from build123d import *

# Parameters (mm, degrees)
SKETCH1_R           = 11
SKETCH1_R_2         = 1.25
BOSS_EXTRUDE1_DEPTH = 3.175


with BuildPart() as part:
    # Sketch1 → Boss-Extrude1 (new body)
    with BuildSketch(Plane(origin=(0, 0, 0), x_dir=(0, 0, -1), z_dir=(1, 0, 0))):
        Circle(SKETCH1_R)
        with BuildLine():
            Line((-2.5, -1.658312395), (-2.5, 1.658312395))
            ThreePointArc((-2.5, 1.658312395), (0.866025404, 2.872281323), (3, 0))
            ThreePointArc((3, 0), (0.866025404, -2.872281323), (-2.5, -1.658312395))
        make_face(mode=Mode.SUBTRACT)
        with Locations((-8, 0)):
            Circle(SKETCH1_R_2, mode=Mode.SUBTRACT)
        with Locations((8, 0)):
            Circle(SKETCH1_R_2, mode=Mode.SUBTRACT)
    extrude(amount=BOSS_EXTRUDE1_DEPTH)


solid = part.part
The model under review builds one solid part; all positions refer to its coordinate system, in mm. Round coordinates to 2 decimals unless told otherwise and drop trailing zeros. Order: outer loops, then holes, each group sorted by start corner. A loop starts at its lowest first (then second) coordinate and runs counter-clockwise, first axis right, second up. Notation, with made-up numbers: (67, 71) -> (77, 71) arc R26 cw to (77, 93) -> close; hole circle Ø3 at (-15.75, -6). An arc over 180 degrees is marked (long way). Write item = value, one per line. Start each with the question number.
Item 1: Consider section C-C on z = -8.5. Write out the cut boundary in (x, y) (3 decimals).
Item 2: For line 1 along Z through (x, y) = (1.6, -0.25); line 2 along Y through (x, z) = (0.5, -1); line 3 along Y through (x, z) = (0.7, 8), list the stretches that pass through material, from the lowest coordinate up.
Item 3: Consider section B-B on x = 1.3. Write out the cut boundary in (y, z).
Item 4: Clearance check with flat-ended pins moving along their axes: pin 1 Ø1 at (y, z) = (7, -2.5) entering from -X; pin 2 Ø1.5 at (y, z) = (0, -8) entering from +X. State where each tip first meets the part, or that it passes through.
Item 5: Consider section A-A on z = 0. Write out the cut boundary in (x, y) (3 decimals).
Item 6: Mouldability with a two-part tool opening along Z and no side actions: class faces 1 (the face through (3.175, 0, 3)), 2 (the face through (2, 0, 2.5)), 3 (the face through (1.57, -10.74, 2.38)) as released by +Z, released by -Z, zero draft, split by the parting line, or undercut.
Conclusion:
q1.outline = (0, -6.982) -> (3.175, -6.982) -> (3.175, -1.146) -> (0, -1.146) -> close; (0, 1.146) -> (3.175, 1.146) -> (3.175, 6.982) -> (0, 6.982) -> close
q2.line_1 = -11 to -9.22, -6.78 to -2.99, 2.5 to 6.78, 9.22 to 11
q2.line_2 = -10.95 to -2.83, 2.83 to 10.95
q2.line_3 = -7.55 to -1.25, 1.25 to 7.55
q3.outline = circle Ø22 at (0, 0); hole (-1.66, 2.5) arc R3 ccw (long way) to (1.66, 2.5) -> close; hole circle Ø2.5 at (0, -8); hole circle Ø2.5 at (0, 8)
q4.pin_1 = 0
q4.pin_2 = through
q5.outline = (0, -11) -> (3.175, -11) -> (3.175, -3) -> (0, -3) -> close; (0, 3) -> (3.175, 3) -> (3.175, 11) -> (0, 11) -> close
q6.face_1 = zero draft
q6.face_2 = undercut
q6.face_3 = split by the parting line
